Can you work these out from the model? Positions are in its coordinate system, mm. Face numbers are marked on the shaded views. A direction names the side the tool comes from. Coordinates: 2 decimals unless noted, no trailing zeros. Loops run counter-clockwise (first coordinate to the right, second up) from the corner with the lowest first, then second, coordinate; pieces in that order, holes last.
```python
from build123d import *

# Parameters (mm, degrees)
F1_DEPTH = 10
F2_R     = 1
F3_R     = 1
F4_R     = 1
F5_W     = 12
F5_H     = 10
F6_DEPTH = 10
F7_W     = 6
F7_H     = 4
F8_DEPTH = 25


with BuildPart() as f1:
    # F0 (on Top) → F1 (new body)
    with BuildSketch(Plane.XY):
        with BuildLine():
            Line((-11.3350533053, 9.1202929616), (-22.3157362798, 9.1202929616))
            Line((-22.3157362798, 9.1202929616), (-22.3157362798, -10))
            Line((-22.3157362798, -10), (-11.3272070885, -10))
            Line((-11.3272070885, -10), (-11.3272070885, -5.2500292659))
            Line((-11.3272070885, -5.2500292659), (-5.7124928571, -5.2500292659))
            Line((-5.7124928571, -5.2500292659), (-5.7124928571, 0.7569257868))
            Line((-5.7124928571, 0.7569257868), (-11.560020037, 0.7569257868))
            Line((-11.560020037, 0.7569257868), (-11.560020037, 2.7420271654))
            Line((-11.560020037, 2.7420271654), (-3.565690713, 2.7420271654))
            Line((-3.565690713, 2.7420271654), (-3.565690713, -10))
            Line((-3.565690713, -10), (6.0123503208, -10))
            Line((6.0123503208, -10), (6.0123503208, 2.7420271654))
            Line((6.0123503208, 2.7420271654), (8.6545692757, 2.7420271654))
            ThreePointArc((8.6545692757, 2.7420271654), (8.5676927282, -1.911451746), (10.2760922164, -6.2408610247))
            ThreePointArc((10.2760922164, -6.2408610247), (13.6839247097, -8.9288594524), (17.8900292945, -10))
            Line((17.8900292945, -10), (18.7280271202, -10))
            Line((18.7280271202, -10), (20.8180968398, -10))
            Line((20.8180968398, -10), (27.6842637202, -8.2088258604))
            Line((27.6842637202, -8.2088258604), (27.6842637202, -2.3396474093))
            Line((27.6842637202, -2.3396474093), (23.8473247737, -3.5986430012))
            Line((23.8473247737, -3.5986430012), (21.4528143406, -3.5986430012))
            ThreePointArc((21.4528143406, -3.5986430012), (19.3461607597, -3.0392900389), (18.4803195298, -1.038994058))
            ThreePointArc((18.4803195298, -1.038994058), (19.2595578745, 1.248700369), (21.4528143406, 2.2637788206))
            Line((21.4528143406, 2.2637788206), (24.837708557, 2.3617743547))
            Line((24.837708557, 2.3617743547), (27.6842637202, 1.6806415132))
            Line((27.6842637202, 1.6806415132), (27.6842637202, 1.6911900602))
            Line((27.6842637202, 1.6911900602), (23.953304423, 8.5980716969))
            ThreePointArc((23.953304423, 8.5980716969), (22.975945626, 8.8371730757), (22.0104184033, 9.1202929616))
            Line((22.0104184033, 9.1202929616), (16.5817085654, 9.1202929616))
            ThreePointArc((16.5817085654, 9.1202929616), (13.4167991013, 8.2553236841), (10.7552717232, 6.3367054882))
            Line((10.7552717232, 6.3367054882), (9.8750670095, 5.1085127981))
            Line((9.8750670095, 5.1085127981), (5.4812123415, 9.1202929616))
            Line((5.4812123415, 9.1202929616), (-7.7649741434, 9.1202929616))
            Line((-7.7649741434, 9.1202929616), (-7.7649741434, 6.2196037167))
            Line((-7.7649741434, 6.2196037167), (-11.3350533053, 9.1202929616))
        make_face()
    extrude(amount=F1_DEPTH)

    # F2
    f2_edges = [f1.edges().sort_by_distance(p)[0] for p in [
        (23.953304, 8.598072, 5),
        (22.010418, 9.120293, 5),
    ]]
    fillet(f2_edges, radius=F2_R)

    # F3
    f3_edges = [f1.edges().sort_by_distance(p)[0] for p in [
        (17.890029, -10, 5),
        (20.818097, -10, 5),
    ]]
    fillet(f3_edges, radius=F3_R)

    # F4
    f4_edges = [f1.edges().sort_by_distance(p)[0] for p in [
        (27.684264, -8.208826, 5),
        (10.276092, -6.240861, 5),
    ]]
    fillet(f4_edges, radius=F4_R)

    # F5 (on face) → F6 (join)
    with BuildSketch(Plane(origin=(-22.3157362798, 0, 0), x_dir=(0, -1, 0), z_dir=(-1, 0, 0))):
        with Locations((0.5, 5)):
            Rectangle(F5_W, F5_H)
    extrude(amount=F6_DEPTH)

    # F7 (on face) → F8 (cut)
    with BuildSketch(Plane.XY.offset(10)):
        with Locations((-25.3084501922, -0.5)):
            Rectangle(F7_W, F7_H)
    extrude(amount=-F8_DEPTH, mode=Mode.SUBTRACT)


solid = f1.part
```
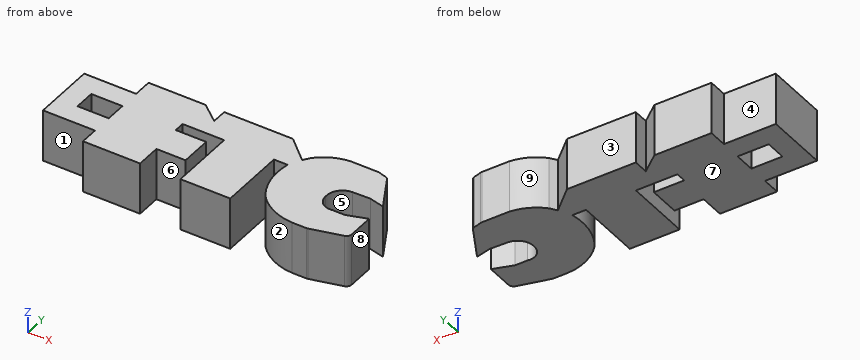
Item 1: I'm going to push flat-ended pins straight in: P1, Ø0.7, axis at x = 22.5, z = 6, coming from the +Y side; P2, Ø3, axis at x = -24, z = 4, coming from the +Y side; P3, Ø3, axis at x = -25, z = 4, coming from the -Y side. Where does each tip first touch, or does it pass through?
Results are:
P1: stops at y = 9.08
P2: stops at y = 5.5
P3: stops at y = -6.5
Item 2: I need wall thicknesses on line 1 along X through (y, z) = (-7.5, 1); line 2 along X through (y, z) = (-0.25, 5.25); line 3 along X through (y, z) = (1, 9). Which ranges of each line are inside material? Lowest first, please.
Results are:
line 1: x = -22.32 to -11.33, -3.57 to 6.01, 11.52 to 27.68
line 2: x = -32.32 to -28.31, -22.31 to -5.71, -3.57 to 6.01, 8.39 to 18.52
line 3: x = -32.32 to -28.31, -22.31 to -11.56, -3.57 to 6.01, 8.41 to 19.06
Item 3: Suppose I cut it at A-A, the plane y = -4.25. Please give me the cut outline in (x, z), plus the area to 3 significant figures.
Results are:
outline: (-32.32, 0) - (-5.71, 0) - (-5.71, 10) - (-32.32, 10) - close; (-3.57, 0) - (6.01, 0) - (6.01, 10) - (-3.57, 10) - close; (9.24, 0) - (27.68, 0) - (27.68, 10) - (9.24, 10) - close
area: 546 mm2
Item 4: We'd pull the mould along X, two halves only. Please class the marked faces 6, 7, 8 and 9: +X half, -X half, draft (parallel to the pull), parting line (faces both ways), or undercut.
Results are:
face 6: undercut
face 7: draft
face 8: +X half
face 9: undercut
Item 5: Suppose I cut it at B-B, the plane x = 7. Please give me the cut outline in (y, z).
Results are:
outline: (2.74, 0) - (7.73, 0) - (7.73, 10) - (2.74, 10) - close
Item 6: On a 3-axis mill with a long thin cutter (end or side, diameter ignored), from which of +Z, -Z, +X, -X, +Y, -Y can I reach the whole of each face in a straight line? I mean the marked faces 1, 2, 3, 4 and 5. Say none if no direction works.
Results are:
face 1: +Z, -Z, -X, -Y
face 2: +Z, -Z, -Y
face 3: +Z, -Z, +X, -X, +Y
face 4: +Z, -Z, -X, +Y
face 5: +Z, -Z
